Geometry check sheet. Reference: drawing and pictorial views, mm from the part's lowest x, y, z. A direction names the side the tool comes from. Give positions to 0.01 mm unless a question says otherwise; leave off trailing zeros. Order: outer loops, then holes, each group sorted by start corner. A loop starts at its lowest first (then second) coordinate and runs counter-clockwise, first axis right, second up.
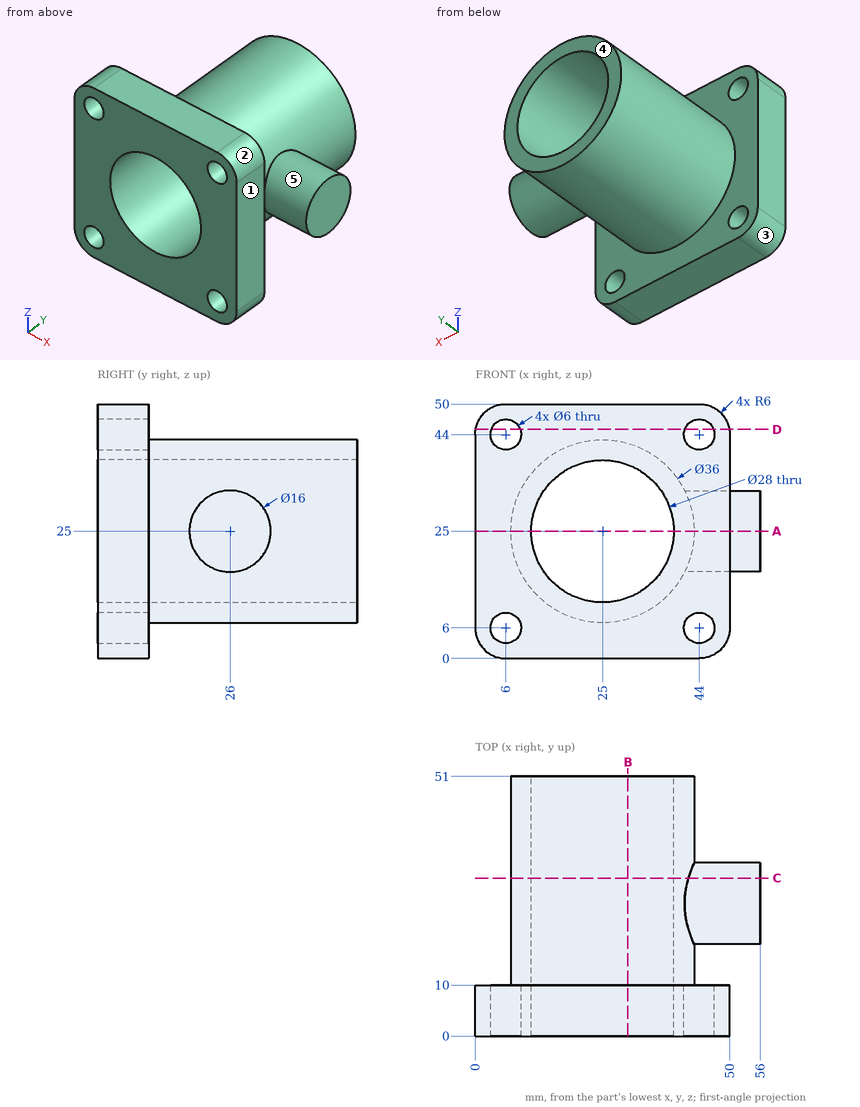
(1) Go/stop test with flat-tipped pins: P1, Ø12, axis at x = 30, y = 18.5, coming from the -Z side; P2, Ø1, axis at y = 27.5, z = 40.5, coming from the -X side; P3, Ø8, axis at x = 14.5, y = 32.5, coming from the -Z side; P4, Ø4, axis at x = 37, y = 11.5, coming from the -Z side. Record where each tip stops, or that it passes through.
(2) Thickness scan on L1, parallel to X at y = 5.75, z = 44; L2, parallel to X at y = 19, z = 25; L3, parallel to X at y = 16, z = 25. Record the ranges inside material, lowest first.
(3) Sectioned sample at D-D (z = 45). Enter the section's corners in (x, y), plus the area to 3 significant figures.
(4) Sectioned sample at A-A (z = 25). Enter the section's corners in (x, y).
(5) Sectioned sample at B-B (x = 30). Enter the section's corners in (y, z), plus the area to 3 significant figures.
(6) Tool access check on the marked faces 1 and 2. Record the directions out of +Z, -Z, +X, -X, +Y, -Y that give a thin tool (end or side, any length) a straight path to the whole face; none if there is none.
(7) Release check for a two-part mould opening along Y. For the marked faces 3, 4 and 5 record: released by +Y, released by -Y, zero draft, split by the parting line, or undercut.
(8) Sectioned sample at C-C (y = 31). Enter the section's corners in (x, z) (3 decimals).
Values follow:
1. P1: stops at z = 7
1. P2: stops at x = 15.05
1. P3: stops at z = 8.21
1. P4: stops at z = 0
2. L1: x = 0 to 3, 9 to 41, 47 to 50
2. L2: x = 7 to 11, 39 to 56
2. L3: x = 7 to 11, 39 to 43
3. outline: (0.08, 0) - (3.17, 0) - (3.17, 10) - (0.08, 10) - close; (8.83, 0) - (41.17, 0) - (41.17, 10) - (8.83, 10) - close; (46.83, 0) - (49.92, 0) - (49.92, 10) - (46.83, 10) - close
3. area: 385 mm2
4. outline: (0, 0) - (11, 0) - (11, 51) - (7, 51) - (7, 10) - (0, 10) - close; (39, 0) - (50, 0) - (50, 10) - (43, 10) - (43, 18) - (56, 18) - (56, 34) - (43, 34) - (43, 51) - (39, 51) - close
5. outline: (0, 0) - (10, 0) - (10, 7.71) - (51, 7.71) - (51, 11.92) - (0, 11.92) - close; (0, 38.08) - (51, 38.08) - (51, 42.29) - (10, 42.29) - (10, 50) - (0, 50) - close
5. area: 584 mm2
6. face 1: +Z, -Z, +X, -Y
6. face 2: +Z, +X, +Y, -Y
7. face 3: zero draft
7. face 4: released by +Y
7. face 5: undercut
8. outline: (41.882, 18.755) - (56, 18.755) - (56, 31.245) - (41.882, 31.245) arc R18 ccw (long way) to start; hole circle Ø28 at (25, 25)
